The listing builds one solid part. Answer for the finished solid, in the listing's coordinates (mm). A direction names the side the tool comes from. Coordinates: 2 decimals unless noted, no trailing zeros. Order: outer loops, then holes, each group sorted by start corner. A loop starts at its lowest first (then second) coordinate and runs counter-clockwise, first axis right, second up.
from build123d import *

# Parameters (mm, degrees)
SKETCH1_W           = 80
SKETCH1_H           = 21.5
BOSS_EXTRUDE1_DEPTH = 6
SKETCH2_W           = 80
SKETCH2_H           = 28
BOSS_EXTRUDE2_DEPTH = 15
SKETCH3_W           = 80
SKETCH3_H           = 22
CUT_EXTRUDE1_DEPTH  = 5
CUT_EXTRUDE2_REACH  = 85.887
SKETCH4_W           = 23.48673248
SKETCH4_H           = 6.968727305


with BuildPart() as part:
    # Sketch1 → Boss-Extrude1 (new body)
    with BuildSketch(Plane(origin=(0, 0, 0), x_dir=(1, 0, 0), z_dir=(0, 1, 0))):
        Rectangle(SKETCH1_W, SKETCH1_H)
    extrude(amount=BOSS_EXTRUDE1_DEPTH)

    # Sketch2 → Boss-Extrude2 (add)
    with BuildSketch(Plane(origin=(0, 6, 0), x_dir=(1, 0, 0), z_dir=(0, 1, 0))):
        Rectangle(SKETCH2_W, SKETCH2_H)
    extrude(amount=BOSS_EXTRUDE2_DEPTH)

    # Sketch3 → Cut-Extrude1 (cut)
    with BuildSketch(Plane(origin=(0, 21, 0), x_dir=(1, 0, 0), z_dir=(0, 1, 0))):
        Rectangle(SKETCH3_W, SKETCH3_H)
    extrude(amount=-CUT_EXTRUDE1_DEPTH, mode=Mode.SUBTRACT)

    # Sketch4 → Cut-Extrude2 (cut, up to next)
    with BuildSketch(Plane(origin=(40, 0, 0), x_dir=(0, 0, -1), z_dir=(1, 0, 0)), mode=Mode.PRIVATE) as cut_extrude2_sk1:
        with Locations((0, 10.569687274)):
            Rectangle(SKETCH4_W, SKETCH4_H)
    cut_extrude2_tool1 = extrude(cut_extrude2_sk1.sketch, amount=-CUT_EXTRUDE2_REACH, mode=Mode.PRIVATE) & part.part
    add(cut_extrude2_tool1.solids().sort_by_distance((40, 10.569687, 0))[0], mode=Mode.SUBTRACT)


solid = part.part
1) Section A-A (y = 11.75) is taken. Give the vertices of the cut face in (x, z).
2) Section B-B (z = -9) is taken. Give the vertices of the cut face in (x, y).
3) Section C-C (x = -32) is taken. Give the vertices of the cut face in (y, z).
4) Section D-D (y = 4.5) is taken. Give the vertices of the cut face in (x, z), then the cut area to 3 significant figures.
5) Consider L1, parallel to Z at x = -22, y = 8; L2, parallel to Y at x = -3, z = 0; L3, parallel to Z at x = -13, y = 18.5. Determine where each line is inside the solid, lowest interval first.
6) Each of these flat-tipped pins is pushed along its axis until it touches: P1, Ø1.8, axis at x = 4.5, y = 3, coming from the +Z side; P2, Ø1, axis at x = 16, z = -12, coming from the -Y side; P3, Ø3, axis at x = 6, y = 4, coming from the -Z side; P4, Ø1.5, axis at y = 18, z = -2.5, coming from the +X side. Where does it stop, or does it pass through?
7) Determine the mould class of faces 5 (the face through (1, 14.054, 0)), 6 (the face through (-1, 16, 0)), 7 (the face through (-1, 13, -14)), 8 (the face through (1, 11, -11.743)) for opening direction Y: released by +Y, released by -Y, zero draft, split by the parting line, or undercut.
8) A tool of negligible diameter and unlimited length cuts with its end or side. For faces 1 (the face through (-1, 6, -12)), 2 (the face through (1, 11, 11.743)), 3 (the face through (-1, 19, -11)), 4 (the face through (-1, 6, 12)), from which of +Z, -Z, +X, -X, +Y, -Y can it reach the whole face along a straight path? Write none if from no direction.
Filled sheet:
1. outline: (-40, -14) - (40, -14) - (40, -11.74) - (-40, -11.74) - close; (-40, 11.74) - (40, 11.74) - (40, 14) - (-40, 14) - close
2. outline: (-40, 0) - (40, 0) - (40, 7.09) - (-40, 7.09) - close; (-40, 14.05) - (40, 14.05) - (40, 16) - (-40, 16) - close
3. outline: (0, -10.75) - (6, -10.75) - (6, -14) - (21, -14) - (21, -11) - (16, -11) - (16, 11) - (21, 11) - (21, 14) - (6, 14) - (6, 10.75) - (0, 10.75) - close; hole (7.09, -11.74) - (14.05, -11.74) - (14.05, 11.74) - (7.09, 11.74) - close
4. outline: (-40, -10.75) - (40, -10.75) - (40, 10.75) - (-40, 10.75) - close
4. area: 1,720 mm2
5. L1: z = -14 to -11.74, 11.74 to 14
5. L2: y = 0 to 7.09, 14.05 to 16
5. L3: z = -14 to -11, 11 to 14
6. P1: stops at z = 10.75
6. P2: stops at y = 6
6. P3: stops at z = -10.75
6. P4: passes through
7. face 5: undercut
7. face 6: released by +Y
7. face 7: zero draft
7. face 8: undercut
8. face 1: -Z, +X, -X, -Y
8. face 2: +X, -X
8. face 3: +X, -X, +Y
8. face 4: +Z, +X, -X, -Y
